Build history of the part. All positions in model axes, mm. Face numbers are marked on the shaded views. A direction names the side the tool comes from. Round coordinates to 2 decimals unless told otherwise and drop trailing zeros. Write each loop counter-clockwise with the first axis right and the second up, starting at its lowest first coordinate (ties: lowest second). Pieces come first, ordered by that corner, then holes. Notation, with made-up numbers: (-8, 46.25) -> (21, 46.25) arc R26 cw to (21, 74.25) -> close; hole circle Ø11 at (67.25, -15.5). An arc over 180 degrees is marked (long way). Answer as CSV lines item,"result".
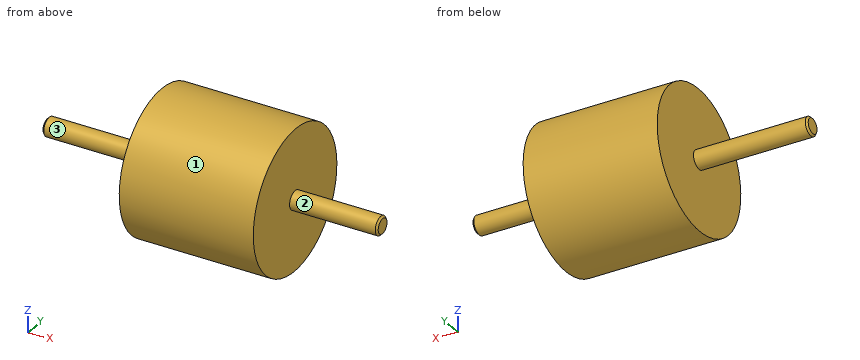
from build123d import *

# Parameters (mm, degrees)
CHANFREIN1_SIZE = 0.5


with BuildPart() as part:
    # Esquisse1 → Révolution1 (revolve)
    with BuildSketch(Plane.XY, mode=Mode.PRIVATE) as r_volution1_sk:
        Polygon((-33.336541, -19.392259), (2.663459, -19.392259), (2.663459, -35.892259), (26.163459, -35.892259), (26.163459, -38.392259), (-63.836541, -38.392259), (-63.836541, -35.892259), (-33.336541, -35.892259), align=None)
    revolve(r_volution1_sk.sketch.rotate(Axis((-107.151340206, -38.392259, 0), (1, 0, 0)), 90), axis=Axis((-107.151340206, -38.392259, 0), (1, 0, 0)))  # turned: the seam where the file's is

    # Chanfrein1
    chanfrein1_edges = [part.edges().sort_by_distance(p)[0] for p in [
        (26.163459, -38.392259, -2.5),
        (-63.836541, -38.392259, -2.5),
    ]]
    chamfer(chanfrein1_edges, length=CHANFREIN1_SIZE)


solid = part.part
1. Cut at D-D, the plane y = -52. Write the cut outline in (x, z).
Results found:
outline,"(-33.34, -13.26) -> (2.66, -13.26) -> (2.66, 13.26) -> (-33.34, 13.26) -> close"
2. Probe line 1 along X through (y, z) = (-42.5, -10.5); line 2 along Z through (x, y) = (-33, -38.5); line 3 along Z through (x, y) = (-25, -21.5). List the from-to ranges inside material, lowest first.
Results found:
line 1,"x = -33.34 to 2.66"
line 2,"z = -19 to 19"
line 3,"z = -8.7 to 8.7"
3. Drop flat-ended pins along their axis: pin 1 Ø5 at (x, z) = (-21.5, 12.5) entering from -Y; pin 2 Ø5 at (x, y) = (9, -41) entering from -Z; pin 3 Ø4 at (x, z) = (-9.5, 5.5) entering from +Y. Give the stop position or say it passes through.
Results found:
pin 1,"stops at y = -54.55"
pin 2,"stops at z = -2.5"
pin 3,"stops at y = -19.72"
4. Cut at A-A, the plane z = 0. Write the cut outline in (x, y), then the cut area to 3 significant figures.
Results found:
outline,"(-63.84, -40.39) -> (-63.34, -40.89) -> (-33.34, -40.89) -> (-33.34, -57.39) -> (2.66, -57.39) -> (2.66, -40.89) -> (25.66, -40.89) -> (26.16, -40.39) -> (26.16, -36.39) -> (25.66, -35.89) -> (2.66, -35.89) -> (2.66, -19.39) -> (-33.34, -19.39) -> (-33.34, -35.89) -> (-63.34, -35.89) -> (-63.84, -36.39) -> close"
area,"1,640 mm2"
5. Cut at B-B, the plane x = -37.5. Write the cut outline in (y, z), then the cut area to 3 significant figures.
Results found:
outline,"circle Ø5 at (-38.39, 0)"
area,"19.6 mm2"
6. Cut at C-C, the plane y = -34. Write the cut outline in (x, z), then the cut area to 3 significant figures.
Results found:
outline,"(-33.34, -18.49) -> (2.66, -18.49) -> (2.66, 18.49) -> (-33.34, 18.49) -> close"
area,"1,330 mm2"
7. Which spindle directions (+Z, -Z, +X, -X, +Y, -Y) get a long thin tool onto all of the face, cutting with end or side? Do the marked faces 1, 2 and 3. Say none if no direction does.
Results found:
face 1,"+X, -X"
face 2,"+X"
face 3,"-X"
